Source: CAD feature listing. Evaluate the final solid. Frame: model axes, mm. A direction names the side the tool comes from. Round coordinates to 2 decimals unless told otherwise and drop trailing zeros. Order: outer loops, then holes, each group sorted by start corner. A loop starts at its lowest first (then second) coordinate and runs counter-clockwise, first axis right, second up. Notation, with made-up numbers: M 28.25,13 L 63.25,13 A18 ccw 63.25,46 Z; hole C -0.75,61 d11. An arc over 180 degrees is marked long. Answer as CSV lines item,"result". Start each with the question number.
Item 1: Line query: line 1 (Z direction, x = 0, y = 2.3); line 2 (X direction, y = 2.7, z = -17.5); line 3 (Z direction, x = 37.5, y = 1.3). Output: solid intervals per line, ascending. Write a range as [from, to].
Item 2: Section query D-D on x = 35.5. Return the cut outline in (y, z).
Item 3: First-contact query: P1, Ø1, axis at x = -13, y = 2, coming from the +Z side; P2, Ø1.6, axis at y = 2.5, z = -22, coming from the -X side; P3, Ø1, axis at x = 42, y = 2, coming from the -Z side; P4, Ø11.5, axis at x = 0, z = 0, coming from the -Y side. Flat tips, straight axial feed; report the tip coordinate or a pass-through.
Item 4: Section query A-A on x = 0. Return the cut outline in (y, z).
Item 5: Section query B-B on z = 0. Return the cut outline in (x, y).
Item 6: Set-up query: faces 1 (the face through (-5, 2, -22)), 2 (the face through (25, 2, -22)), 3 (the face through (-5, 2, 22)), 4 (the face through (25, 2, 22)). Return all of +Z, -Z, +X, -X, +Y, -Y with unobstructed straight access to the full face (end or side cutting, diameter ignored); none if empty.
Item 7: Pull-direction query (Z, two-part tool) for faces 5 (the face through (-12, 2, -20)), 6 (the face through (-13, 2, 20)), 7 (the face through (-4.38, 1.57, 8.43)); classes: +Z half, -Z half, draft (parallel to the pull), parting line (faces both ways), or undercut.
Item 8: Section query C-C on y = 2.6. Return the cut outline in (x, z), plus the area to 3 significant figures.
Autodesk Inventor part; units mm, degrees
ref_plane "YZ Plane" through (0, 0, 0) normal (1, 0, 0) x (0, 1, 0)
ref_plane "XZ Plane" through (0, 0, 0) normal (0, 1, 0) x (-1, 0, 0)
ref_plane "XY Plane" through (0, 0, 0) normal (0, 0, 1) x (1, 0, 0)
sketch "Boceto1" plane through (0, 0, 0) normal (0, 1, 0) x (-1, 0, 0)
  circle A0 centre (0, 0) radius 9.5
  line L0 (20, 20) -> (-40, 20)
  line L1 (-40, 20) -> (-40, -20)
  line L2 (-40, -20) -> (20, -20)
  line L3 (20, -20) -> (20, 20)
  line L4 (5, 23.18) -> (-25, 23.18)
  line L5 (-25, 23.18) -> (-25, 20)
  line L6 (-25, 20) -> (5, 20)
  line L7 (5, 20) -> (5, 23.18)
  line L8 (5, -20) -> (-25, -20)
  line L9 (-25, -20) -> (-25, -23.18)
  line L10 (-25, -23.18) -> (5, -23.18)
  line L11 (5, -23.18) -> (5, -20)
  line L12 (-40, 10) -> (-43.18, 10)
  line L13 (-43.18, 10) -> (-43.18, -10)
  line L14 (-43.18, -10) -> (-40, -10)
  line L15 (-40, -10) -> (-40, 10)
  dimension "d0" = 19
  dimension "d17" = 40
  dimension "d18" = 60
  dimension "d19" = 20
  dimension "d20" = 20
  dimension "d21" = 3.18
  dimension "d22" = 30
  dimension "d23" = 15
  dimension "d24" = 20
  dimension "d25" = 10
  dimension "d26" = 3.18
extrude "Extrusión1" add sketch "Boceto1" along normal blind 3.18
properties part number "HOMBRO_SOST.COJ"
Results:
1,line 1,"[-23.18, -9.5], [9.5, 23.18]"
1,line 2,"[-20, 40]"
1,line 3,"[-20, 20]"
2,outline,"M 0,-20 L 3.18,-20 L 3.18,20 L 0,20 Z"
3,P1,"z = 20"
3,P2,"x = -5"
3,P3,"z = -10"
3,P4,"through"
4,outline,"M 0,-23.18 L 3.18,-23.18 L 3.18,-9.5 L 0,-9.5 Z; M 0,9.5 L 3.18,9.5 L 3.18,23.18 L 0,23.18 Z"
5,outline,"M -20,0 L -9.5,0 L -9.5,3.18 L -20,3.18 Z; M 9.5,0 L 43.18,0 L 43.18,3.18 L 9.5,3.18 Z"
6,face 1,"-Z, -X, +Y, -Y"
6,face 2,"-Z, +X, +Y, -Y"
6,face 3,"+Z, -X, +Y, -Y"
6,face 4,"+Z, +X, +Y, -Y"
7,face 5,"-Z half"
7,face 6,"+Z half"
7,face 7,"undercut"
8,outline,"M -20,-20 L -5,-20 L -5,-23.18 L 25,-23.18 L 25,-20 L 40,-20 L 40,-10 L 43.18,-10 L 43.18,10 L 40,10 L 40,20 L 25,20 L 25,23.18 L -5,23.18 L -5,20 L -20,20 Z; hole C 0,0 d19"
8,area,"2,370 mm^2"
